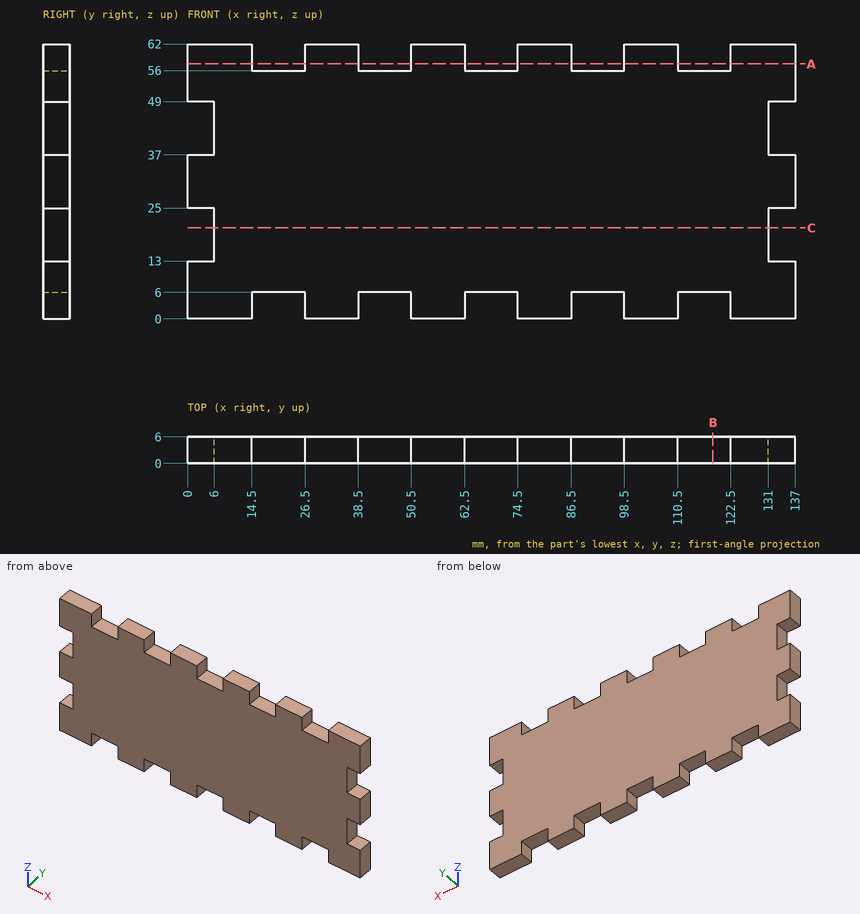
Could you check a few things on this drawing? It's one solid part, dimensions in mm from its lowest x, y, z. Round coordinates to 2 decimals unless told otherwise and drop trailing zeros. Order: outer loops, then holes, each group sorted by start corner. A loop starts at its lowest first (then second) coordinate and runs counter-clockwise, first axis right, second up. Notation, with made-up numbers: M 72,-13.5 L 97,-13.5 A16 ccw 97,-5.5 Z; hole C -9.75,-4.5 d2. An arc over 180 degrees is marked long. One line per item, written item: value.
(1) Imagine slicing it at A-A (z = 57.5). Write out the boundary of the cut face in (x, y), and give its area (3 significant figures).
Ans:
outline: M 0,0 L 14.5,0 L 14.5,6 L 0,6 Z; M 26.5,0 L 38.5,0 L 38.5,6 L 26.5,6 Z; M 50.5,0 L 62.5,0 L 62.5,6 L 50.5,6 Z; M 74.5,0 L 86.5,0 L 86.5,6 L 74.5,6 Z; M 98.5,0 L 110.5,0 L 110.5,6 L 98.5,6 Z; M 122.5,0 L 137,0 L 137,6 L 122.5,6 Z
area: 462 mm^2
(2) Imagine slicing it at B-B (x = 118.5). Write out the boundary of the cut face in (y, z).
Ans:
outline: M 0,6 L 6,6 L 6,56 L 0,56 Z
(3) Imagine slicing it at C-C (z = 20.5). Write out the boundary of the cut face in (x, y).
Ans:
outline: M 6,0 L 131,0 L 131,6 L 6,6 Z
(4) I need wall thicknesses on line 1 along X through (y, z) = (0.8, 4.5); line 2 along Z through (x, y) = (20.5, 5.55); line 3 along X through (y, z) = (2.2, 17.5). Which ranges of each line are inside material? Lowest first, please. Write a range as from..to.
Ans:
line 1: x = 0..14.5, 26.5..38.5, 50.5..62.5, 74.5..86.5, 98.5..110.5, 122.5..137
line 2: z = 6..56
line 3: x = 6..131
(5) I'm going to push flat-ended pins straight in: P1, Ø3, axis at x = 20, y = 4, coming from the +Z side; P2, Ø3, axis at y = 3, z = 18, coming from the -X side. Where does each tip first touch, or does it pass through?
Ans:
P1: stops at z = 56
P2: stops at x = 6
